Autodesk Fusion 360 part; units mm, degrees
sketch "Sketch1" plane through (0, 0, 0) normal (0, 1, 0) x (1, 0, 0) in component "Box"
  line L0 (0, 0) -> (80, 0)
  line L1 (80, 0) -> (80, -60)
  line L2 (80, -60) -> (0, -60)
  line L3 (0, -60) -> (0, 0)
  dimension "d1" = 60
  dimension "d2" = 80
extrude "Extrude1" add sketch "Sketch1" along normal blind 47.5 in component "Box"
sketch "Sketch2" plane through (0, 0, 0) normal (0, 1, 0) x (1, 0, 0) in component "Box"
  line L0 (75, -5) -> (5, -5)
  line L1 (5, -5) -> (5, -55)
  line L2 (5, -55) -> (75, -55)
  line L3 (75, -55) -> (75, -5)
  line L4 (75, -5) -> (5, -55) construction
  line L5 (5, -5) -> (75, -55) construction
  line L6 (0, 0) -> (0, -60)
  point P0 (40, -30)
  point P1 (80, 0)
  point P2 (80, -60)
  dimension "d5" = 70
  dimension "d6" = 50
  dimension "d7" = 60
  dimension "d8" = 60
extrude "Extrude2" cut sketch "Sketch2" along normal blind 45 in component "Box"
fillet "Fillet1" radius 2.5 2 edges at (0, 23.75, 60) (0, 23.75, 0) in component "Box"
fillet "Fillet2" radius 2.5 2 edges at (80, 23.75, 60) (80, 23.75, 0) in component "Box"
sketch "Sketch3" plane through (0, 0, 0) normal (-1, 0, 0) x (0, -1, 0) in component "Box"
  line L0 (-47.5, 2.5) -> (0, 2.5)
  line L1 (0, 2.5) -> (0, 57.5)
  line L2 (0, 57.5) -> (-47.5, 57.5)
  line L3 (-47.5, 57.5) -> (-47.5, 2.5)
  circle A0 centre (-30, 40) radius 13.335
  dimension "d13" = 26.67
extrude "Extrude3" cut sketch "Sketch3" against normal blind 30 contours A0 in component "Box"
delete_face "DeleteFace1" 1 faces at (1.6667, 16.7313, 38.6723) in component "Box"
sketch "Sketch1 (2)" plane through (0, 0, 0) normal (-1, 0, 0) x (0, -1, 0)
  line L0 (-47.5, 2.5) -> (0, 2.5)
  line L1 (0, 2.5) -> (0, 57.5)
  line L2 (0, 57.5) -> (-47.5, 57.5)
  line L3 (-47.5, 57.5) -> (-47.5, 2.5)
  circle A0 centre (-30, 40) radius 13.5
  dimension "d16" = 27
extrude "Extrude4" cut sketch "Sketch1 (2)" against normal blind 50 contours A0 in component "Box"
delete_face "DeleteFace2" 1 faces at (78.4292, 15.8333, 0.1791) in component "Box"
delete_face "DeleteFace3" 1 faces at (77.9731, 15.8333, 59.9548) in component "Box"
extrude "Extrude5" add 1 faces at (80, 15.8333, 20) along direction (1, 0, 0) blind 43.18 in component "Box"
extrude "Extrude6" cut 1 faces at (75, 15, 38.3333) along direction (1, 0, 0) blind 45 in component "Box"
delete_face "DeleteFace4" 1 faces at (0.0028, 15.8333, 2.381) in component "Box"
delete_face "DeleteFace5" 1 faces at (2.381, 15.8333, 59.9972) in component "Box"
extrude "Extrude7" add 1 faces at (41.06, 31.6667, 0) along direction (0, 0, -1) blind 68.58 in component "Box"
extrude "Extrude8" cut 1 faces at (43.3333, 15, 5) along direction (0, 0, -1) blind 70 in component "Box"
extrude "Extrude9" cut 1 faces at (5, 24.6637, -34.4874) along direction (-1, 0, 0) blind 2 in component "Box"
extrude "Extrude10" cut 1 faces at (81, 30, 55) along direction (0, 0, 1) blind 2 in component "Box"
fillet "Fillet3" radius 2.5 1 edges at (123.18, 23.75, -68.58) in component "Box"
fillet "Fillet4" radius 2.5 1 edges at (0, 23.75, -68.58) in component "Box"
fillet "Fillet5" radius 2.5 1 edges at (0, 23.75, 60) in component "Box"
fillet "Fillet6" radius 2.5 1 edges at (123.18, 23.75, 60) in component "Box"
extrude "Extrude11" cut 1 faces at (42, 15, -65) along direction (0, 0, -1) blind 2 in component "Box"
extrude "Extrude12" cut 1 faces at (81, 30, 57) along direction (0, 0, 1) blind 0.15 in component "Box"
extrude "Extrude13" cut 1 faces at (81, 30, 57.15) along direction (0, 0, 1) blind 0.5 in component "Box"
extrude "Extrude14" cut 1 faces at (81, 30, 57.65) along direction (0, 0, 1) blind 0.5 in component "Box"
extrude "Extrude15" cut 1 faces at (120, 15, -25.2833) along direction (1, 0, 0) blind 0.5 in component "Box"
extrude "Extrude16" cut 1 faces at (120.5, 15, -25.2833) along direction (1, 0, 0) blind 0.5 in component "Box"
extrude "Extrude17" cut 1 faces at (121, 15, -25.2833) along direction (1, 0, 0) blind 0.3 in component "Box"
extrude "Extrude18" cut 1 faces at (121.3, 15, -25.2833) along direction (1, 0, 0) blind 0.2 in component "Box"
extrude "Extrude19" cut 1 faces at (3, 24.6637, -35.8208) along direction (-1, 0, 0) blind 2 in component "Box"
extrude "Extrude20" add 1 faces at (1, 24.6637, -35.8208) along direction (1, 0, 0) blind 0.5 in component "Box"
extrude "Extrude21" add 1 faces at (1.5, 24.6637, -35.8208) along direction (1, 0, 0) blind 0.5 in component "Box"
component "Box" placed x (1, 0, 0) y (0, 1, 0) z (0, 0, 1) at (0, 0, 0)
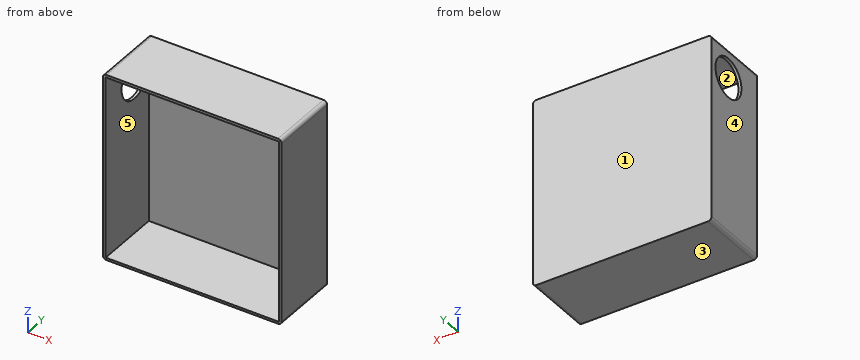
For this review, take the finished solid that the model builds, in its own axes (mm). Face numbers are marked on the shaded views. A direction names the side the tool comes from. Coordinates: 2 decimals unless noted, no trailing zeros. Write each loop counter-clockwise with the first axis right and the second up, starting at its lowest first coordinate (ties: lowest second). Pieces come first, ordered by that corner, then holes. Notation, with made-up numbers: (23, -39) - (33, -39) arc R20 ccw to (33, -8) - close; hole circle Ø1 at (27, 73). An arc over 180 degrees is marked (long way). Answer in a Markdown table with one row per item. Add a question column.
Q1. We need section B-B, the plane y = 30. State the section outline as (x, z) points.
Q2. We need section A-A, the plane z = 40. State the section outline as (x, y) points, and give its area (3 significant figures).
Q3. For probe 1 along X at (y, z) = (7.5, 53.5); probe 2 along Z at (x, y) = (63.5, 21); probe 3 along Y at (x, z) = (27, -38.5), list the stretches that pass through material, from the lowest coordinate up.
Q4. Draft analysis for pull direction Z (two halves, no side actions). For the marked faces 1, 2 and 3, state which applies: +Z half, -Z half, draft (parallel to the pull), parting line (faces both ways), or undercut.
Q5. We need section C-C, the plane x = 75.5. State the section outline as (y, z) points, and give its area (3 significant figures).
Q6. We need section D-D, the plane z = -56.5. State the section outline as (x, y) points.
Q7. Tool access review of the marked faces 4 and 5: name each direction out of +Z, -Z, +X, -X, +Y, -Y from which nothing blocks a thin tool from reaching the whole face with its end or side.
Answer list:
| question | item | result |
|---|---|---|
| 1 | outline | (0, -66.08) arc R2.5 ccw to (2.5, -68.58) - (120.68, -68.58) arc R2.5 ccw to (123.18, -66.08) - (123.18, 57.5) arc R2.5 ccw to (120.68, 60) - (2.5, 60) arc R2.5 ccw to (0, 57.5) - (0, 53.5) - (2, 53.5) - (2, 58.15) - (121.5, 58.15) - (121.5, -67) - (2, -67) - (2, 26.5) - (0, 26.5) - close |
| 2 | outline | (0, 0) - (2, 0) - (2, 16.5) - (0, 16.5) - close; (0, 43.5) - (2, 43.5) - (2, 45) - (121.5, 45) - (121.5, 0) - (123.18, 0) - (123.18, 47.5) - (0, 47.5) - close |
| 2 | area | 420 mm2 |
| 3 | probe 1 | x = 0 to 2, 121.5 to 123.18 |
| 3 | probe 2 | z = -68.58 to -67, 58.15 to 60 |
| 3 | probe 3 | y = 45 to 47.5 |
| 4 | face 1 | draft |
| 4 | face 2 | undercut |
| 4 | face 3 | -Z half |
| 5 | outline | (0, -68.58) - (47.5, -68.58) - (47.5, 60) - (0, 60) - (0, 58.15) - (45, 58.15) - (45, -67) - (0, -67) - close |
| 5 | area | 476 mm2 |
| 6 | outline | (0, 0) - (2, 0) - (2, 45) - (121.5, 45) - (121.5, 0) - (123.18, 0) - (123.18, 47.5) - (0, 47.5) - close |
| 7 | face 4 | +Z, -Z, -X, +Y, -Y |
| 7 | face 5 | -Y |
